```python
from build123d import *

# Parameters (mm, degrees)
CYLINDER008_R              = 4
CYLINDER008_DEPTH          = 620
REVOLVE006_PLACEMENT_ANGLE = 180
CYLINDER009_R              = 5
CYLINDER009_DEPTH          = 30
REVOLVE007_PLACEMENT_ANGLE = 180


with BuildPart() as cylinder008:
    # Cylinder008 → Cylinder008 (new body)
    with BuildSketch(Plane.XY):
        Circle(CYLINDER008_R)
    extrude(amount=CYLINDER008_DEPTH)


with BuildPart() as revolve006:
    # Sketch006 → Revolve006 (revolve)
    with BuildSketch(Plane.XZ):
        Polygon((0, 0), (0, 4), (4, 4), (4, 7), (1, 7), (1, 11.5), (3.5, 11.5), (3.5, 7), (0.5, 7), (0.5, 4), (4.5, 4), (4.5, 0), align=None)
    revolve(axis=Axis((0, 0, 0), (0, 0, 1)))


with BuildPart() as revolve006_1:
    # Revolve006 placement: moved
    add(revolve006.part.rotate(Axis((0, 0, 0), (0, 1, 0)), REVOLVE006_PLACEMENT_ANGLE))


with BuildPart() as cylinder009:
    # Cylinder009 → Cylinder009 (new body)
    with BuildSketch(Plane.XY.offset(618)):
        Circle(CYLINDER009_R)
    extrude(amount=CYLINDER009_DEPTH)


with BuildPart() as straw003:
    # Sketch007 → Revolve007 (revolve)
    with BuildSketch(Plane.YZ):
        Polygon((0, 0), (0, 1), (-0.5, 1), (-0.5, 2.5), (0, 2.5), (0, 5), (-0.5, 5), (-0.5, 6.5), (0, 6.5), (0, 15.5), (6, 15.5), (6, 6.5), (6.5, 6.5), (6.5, 5), (6, 5), (6, 2.5), (6.5, 2.5), (6.5, 1), (6, 1), (6, 0), align=None)
    revolve(axis=Axis((0, 0, 0), (0, 0, 1)))


with BuildPart() as straw003_1:
    # Revolve007 placement: moved
    add(straw003.part.moved(Location((0, 0, 631.5))).rotate(Axis((0, 0, 631.5), (1, 0, 0)), REVOLVE007_PLACEMENT_ANGLE))

    # Cut006: cut Cylinder009
    add(cylinder009.part, mode=Mode.SUBTRACT)

    # Fusion003: union Cylinder008, Revolve006
    add(cylinder008.part)
    add(revolve006_1.part)


with BuildPart() as straw003_2:
    # Fusion003 placement: moved
    add(straw003_1.part.moved(Location((0, 0, -42))))


solid = straw003_2.part
```
CAD build for the part. Positions are in the model's coordinates, mm. A direction names the side the tool comes from. Coordinates: 2 decimals unless noted, no trailing zeros. Write each loop counter-clockwise with the first axis right and the second up, starting at its lowest first coordinate (ties: lowest second). Pieces come first, ordered by that corner, then holes. Notation, with made-up numbers: (-20.5, -28) -> (22.5, -28) arc R32 cw to (22.5, 6) -> close; hole circle Ø8 at (59, 84). An arc over 180 degrees is marked (long way). Use CSV: the item, a comma, the result in double quotes. Start each with the question number.
Item 1: Wall check: probe 1 along Y at (x, z) = (0, 586.5); probe 2 along Z at (x, y) = (3.75, -2.25); probe 3 along Z at (x, y) = (2, -5.75). Give the ranges that are in metal, low to high.
Item 2: Tool access for faces 4 (the cylindrical face through (-1.802, -5.723, 578.563)), 5 (the cylindrical face through (3.955, 5.158, 583.76)), 6 (the flat face through (3.92, -1.42, 574)), 7 (the flat face through (6, -2, 588.5)), 8 (the flat face through (-4, 4, 589.5)): list every direction of +Z, -Z, +X, -X, +Y, -Y with a clear straight run to the whole face (end or side of a thin tool).
Item 3: Drop flat-ended pins along their axis: P1, Ø5, axis at x = -2.5, z = 225, coming from the -Y side; P2, Ø6, axis at x = 0, z = 524.5, coming from the +Y side; P3, Ø4, axis at x = 1, y = -1.5, coming from the +Z side. Give the stop position or say it passes through.
Item 4: Two-plate mould, pull along Y, no slides. Class faces 1 (the cylindrical face through (3.955, 5.158, 587.76)), 2 (the flat face through (6, 2, 583)), 3 (the cylindrical face through (-1.08, -4.88, 582.66)): +Y half, -Y half, draft (parallel to the pull), parting line (faces both ways), or undercut.
Item 5: Band-saw the part on A-A, the plane z = 311. Write the cut outline in (x, y), plus the area to 3 significant figures.
Response values:
1,probe 1,"y = -6 to -5, 5 to 6"
1,probe 2,"z = -46 to -42, 574 to 576"
1,probe 3,"z = 583 to 584.5, 587 to 588.5"
2,face 4,"-Z"
2,face 5,"+Z, -Z"
2,face 6,"none"
2,face 7,"+Z"
2,face 8,"+Z, +X, -X, +Y, -Y"
3,P1,"stops at y = -4"
3,P2,"stops at y = 4"
3,P3,"stops at z = 578"
4,face 1,"parting line"
4,face 2,"draft"
4,face 3,"undercut"
5,outline,"circle Ø8 at (0, 0)"
5,area,"50.3 mm2"
